Design review of the part built by this model. Coordinates are the model's own, in mm. A direction names the side the tool comes from. Coordinates: 2 decimals unless noted, no trailing zeros. Order: outer loops, then holes, each group sorted by start corner. A loop starts at its lowest first (then second) coordinate and runs counter-clockwise, first axis right, second up. Notation, with made-up numbers: M 49,-36.5 L 85,-36.5 A14 ccw 85,-22.5 Z; hole C 65.25,-33.75 d7. An arc over 180 degrees is marked long. Answer as a JSON object with one key per item and string values.
from build123d import *

# Parameters (mm, degrees)
SKETCH1_R           = 2
SKETCH1_R_2         = 3.5
BOSS_EXTRUDE1_DEPTH = 270


with BuildPart() as part:
    # Sketch1 → Boss-Extrude1 (new body)
    with BuildSketch(Plane.XY):
        with BuildLine():
            Line((-5, -3), (-5, 3))
            Line((-5, 3), (-7, 3))
            Line((-7, 3), (-7, 4.298364791))
            Line((-7, 4.298364791), (-13.5, 4.298364791))
            Line((-13.5, 4.298364791), (-13.5, 3))
            Line((-13.5, 3), (-15, 3))
            Line((-15, 3), (-15, 14))
            ThreePointArc((-15, 14), (-14.707106781, 14.707106781), (-14, 15))
            Line((-14, 15), (-3, 15))
            Line((-3, 15), (-3, 13.5))
            Line((-3, 13.5), (-5, 13.5))
            Line((-5, 13.5), (-5, 7))
            Line((-5, 7), (-3, 7))
            Line((-3, 7), (-3, 5))
            Line((-3, 5), (3, 5))
            Line((3, 5), (3, 7))
            Line((3, 7), (5, 7))
            Line((5, 7), (5, 13.5))
            Line((5, 13.5), (3, 13.5))
            Line((3, 13.5), (3, 15))
            Line((3, 15), (27, 15))
            Line((27, 15), (27, 13.5))
            Line((27, 13.5), (25, 13.5))
            Line((25, 13.5), (25, 7))
            Line((25, 7), (27, 7))
            Line((27, 7), (27, 5))
            Line((27, 5), (33, 5))
            Line((33, 5), (33, 7))
            Line((33, 7), (35, 7))
            Line((35, 7), (35, 13.5))
            Line((35, 13.5), (33, 13.5))
            Line((33, 13.5), (33, 15))
            Line((33, 15), (44, 15))
            ThreePointArc((44, 15), (44.707106781, 14.707106781), (45, 14))
            Line((45, 14), (45, 3))
            Line((45, 3), (43.5, 3))
            Line((43.5, 3), (43.5, 4.298364791))
            Line((43.5, 4.298364791), (37, 4.298364791))
            Line((37, 4.298364791), (37, 3))
            Line((37, 3), (35, 3))
            Line((35, 3), (35, -3))
            Line((35, -3), (37, -3))
            Line((37, -3), (37, -4.298364791))
            Line((37, -4.298364791), (43.5, -4.298364791))
            Line((43.5, -4.298364791), (43.5, -3))
            Line((43.5, -3), (45, -3))
            Line((45, -3), (45, -14))
            ThreePointArc((45, -14), (44.707106781, -14.707106781), (44, -15))
            Line((44, -15), (33, -15))
            Line((33, -15), (33, -13.5))
            Line((33, -13.5), (35, -13.5))
            Line((35, -13.5), (35, -7))
            Line((35, -7), (33, -7))
            Line((33, -7), (33, -5))
            Line((33, -5), (27, -5))
            Line((27, -5), (27, -7))
            Line((27, -7), (25, -7))
            Line((25, -7), (25, -13.5))
            Line((25, -13.5), (27, -13.5))
            Line((27, -13.5), (27, -15))
            Line((27, -15), (3, -15))
            Line((3, -15), (3, -13.5))
            Line((3, -13.5), (5, -13.5))
            Line((5, -13.5), (5, -7))
            Line((5, -7), (3, -7))
            Line((3, -7), (3, -5))
            Line((3, -5), (-3, -5))
            Line((-3, -5), (-3, -7))
            Line((-3, -7), (-5, -7))
            Line((-5, -7), (-5, -13.5))
            Line((-5, -13.5), (-3, -13.5))
            Line((-3, -13.5), (-3, -15))
            Line((-3, -15), (-14, -15))
            ThreePointArc((-14, -15), (-14.707106781, -14.707106781), (-15, -14))
            Line((-15, -14), (-15, -3))
            Line((-15, -3), (-13.5, -3))
            Line((-13.5, -3), (-13.5, -4.298364791))
            Line((-13.5, -4.298364791), (-7, -4.298364791))
            Line((-7, -4.298364791), (-7, -3))
            Line((-7, -3), (-5, -3))
        make_face()
        Circle(SKETCH1_R, mode=Mode.SUBTRACT)
        with Locations((-10.606601718, 10.606601718)):
            Circle(SKETCH1_R_2, mode=Mode.SUBTRACT)
        with Locations((40.606601718, 10.606601718)):
            Circle(SKETCH1_R_2, mode=Mode.SUBTRACT)
        with Locations((30, 0)):
            Circle(SKETCH1_R, mode=Mode.SUBTRACT)
        with Locations((40.606601718, -10.606601718)):
            Circle(SKETCH1_R_2, mode=Mode.SUBTRACT)
        with Locations((-10.606601718, -10.606601718)):
            Circle(SKETCH1_R_2, mode=Mode.SUBTRACT)
        with BuildLine():
            Line((4, -3), (4, 3))
            Line((4, 3), (7, 6))
            Line((7, 6), (7, 11))
            ThreePointArc((7, 11), (7.292893219, 11.707106781), (8, 12))
            Line((8, 12), (22, 12))
            ThreePointArc((22, 12), (22.707106781, 11.707106781), (23, 11))
            Line((23, 11), (23, 6))
            Line((23, 6), (26, 3))
            Line((26, 3), (26, -3))
            Line((26, -3), (23, -6))
            Line((23, -6), (23, -11))
            ThreePointArc((23, -11), (22.707106781, -11.707106781), (22, -12))
            Line((22, -12), (8, -12))
            ThreePointArc((8, -12), (7.292893219, -11.707106781), (7, -11))
            Line((7, -11), (7, -6))
            Line((7, -6), (4, -3))
        make_face(mode=Mode.SUBTRACT)
    extrude(amount=BOSS_EXTRUDE1_DEPTH)


solid = part.part
1) Add section C-C (z = 224.5). Count the separate pieces of the cut face and the enclosed holes in it, and give its area (3 significant figures).
Taken from the geometry:
{"separate pieces": "1", "enclosed holes": "7", "area": "685 mm2"}
2) Add section A-A (x = 19.5). State the section outline as (y, z) points.
Taken from the geometry:
{"outline": "M -15,0 L -12,0 L -12,270 L -15,270 Z; M 12,0 L 15,0 L 15,270 L 12,270 Z"}
3) Insertion check: pin 1 Ø2.5 at (x, y) = (30, 0) entering from -Z; pin 2 Ø0.8 at (y, z) = (14.5, 118.5) entering from +X (3 decimals). Each pin has a flat end and moves straight along its axis. Give the tip position at first contact, or say it passes through.
Taken from the geometry:
{"pin 1": "passes through", "pin 2": "stops at x = 44.995"}
4) Tool access review of faces 1 (the flat face through (25, -10, 133)), 2 (the flat face through (-5, 0, 133)), 3 (the flat face through (0, -5, 133)), 4 (the flat face through (0, 5, 133)): name each direction out of +Z, -Z, +X, -X, +Y, -Y from which nothing blocks a thin tool from reaching the whole face with its end or side.
Taken from the geometry:
{"face 1": "+Z, -Z", "face 2": "+Z, -Z, -X", "face 3": "+Z, -Z, -Y", "face 4": "+Z, -Z, +Y"}
5) To check wall thickness, follow L1, parallel to X at y = -11, z = 105.5; L2, parallel to Y at x = 36, z = 140; L3, parallel to X at y = 4, z = 202. State the ranges of each line that lie inside material, in increasing order.
Taken from the geometry:
{"L1": "x = -15 to -14.08, -7.13 to -5, 5 to 7, 23 to 25, 35 to 37.13, 44.08 to 45", "L2": "y = -15 to -3, 3 to 15", "L3": "x = -15 to -13.5, -7 to 5, 25 to 37, 43.5 to 45"}
6) Mouldability with a two-part tool opening along Y and no side actions: class faces 5 (the flat face through (4, 0, 133)), 6 (the flat face through (-15, -9, 133)), 7 (the flat face through (-9, 15, 133)) as released by +Y, released by -Y, zero draft, split by the parting line, or undercut.
Taken from the geometry:
{"face 5": "undercut", "face 6": "zero draft", "face 7": "released by +Y"}
7) Add section B-B (x = 40). State the section outline as (y, z) points, and give its area (3 significant figures).
Taken from the geometry:
{"outline": "M -15,0 L -14.05,0 L -14.05,270 L -15,270 Z; M -7.16,0 L -4.3,0 L -4.3,270 L -7.16,270 Z; M 4.3,0 L 7.16,0 L 7.16,270 L 4.3,270 Z; M 14.05,0 L 15,0 L 15,270 L 14.05,270 Z", "area": "2,060 mm2"}
